Could you check a few things on this model? Use its own coordinates, in mm. A direction names the side the tool comes from. Give positions to 0.01 mm unless a question says otherwise; leave off trailing zeros. Write each loop counter-clockwise with the first axis right and the second up, starting at its lowest first coordinate (ties: lowest second). Pieces come first, ordered by that corner, then holes. Notation, with made-up numbers: (0, -38.5) - (9, -38.5) arc R11 ccw to (9, -26.5) - close; hole circle Ø7 at (-37.75, -24.5). An arc over 180 degrees is marked (long way). Use one line per item in the form item = value.
Autodesk Inventor part; units mm, degrees
ref_plane "YZ Plane" through (0, 0, 0) normal (1, 0, 0) x (0, 1, 0)
ref_plane "XZ Plane" through (0, 0, 0) normal (0, 1, 0) x (-1, 0, 0)
ref_plane "XY Plane" through (0, 0, 0) normal (0, 0, 1) x (1, 0, 0)
sketch "Skizze1" plane through (0, 0, 0) normal (0, 1, 0) x (-1, 0, 0)
  line L0 (0, 0) -> (54.1, 0)
  line L1 (54.1, 0) -> (54.1, -94.74)
  line L2 (54.1, -94.74) -> (0, -94.74)
  line L3 (0, -94.74) -> (0, 0)
  dimension "d0" = 94.74
  dimension "d1" = 54.1
extrude "Extrusion1" add sketch "Skizze1" along normal blind 1.5
sketch "Skizze2" plane through (0, 1.5, 0) normal (0, 1, 0) x (1, 0, 0)
  line L0 (-54.1, 0) -> (0, 0)
  line L1 (0, 94.74) -> (-54.1, 94.74)
  line L2 (0, 0) -> (-54.1, 0)
  line L3 (-54.1, 0) -> (-54.1, 94.74)
  line L4 (-54.1, 94.74) -> (0, 94.74)
  line L5 (0, 94.74) -> (0, 0)
  line L6 (-53.35, 93.99) -> (-53.35, 0.75)
  line L7 (-53.35, 0.75) -> (-0.75, 0.75)
  line L8 (-0.75, 0.75) -> (-0.75, 93.99)
  line L9 (-0.75, 93.99) -> (-53.35, 93.99)
  dimension "d4" = 0.75
extrude "Extrusion2" cut sketch "Skizze2" against normal blind 0.75
sketch "Skizze3" plane through (0, 1.5, 0) normal (0, 1, 0) x (1, 0, 0)
  circle A0 centre (-42.29, 9.27) radius 4
  circle A1 centre (-42.29, 85.47) radius 4
  circle A2 centre (-6.73, 85.47) radius 4
  circle A3 centre (-6.73, 9.27) radius 4
  line L0 (0, 0) -> (-54.1, 0)
  line L1 (-0.75, 0.75) -> (-0.75, 93.99)
  line L2 (-53.35, 0.75) -> (-0.75, 0.75)
  dimension "d7" = 8
  dimension "d8" = 8
  dimension "d9" = 8
  dimension "d10" = 8
  dimension "d12" = 5.98
  dimension "d13" = 5.98
  dimension "d14" = 35.56
  dimension "d15" = 35.56
  dimension "d16" = 8.52
  dimension "d17" = 76.2
extrude "Extrusion3" add sketch "Skizze3" along normal blind 4.25
sketch "Skizze4" plane through (-42.29, 5.75, -9.27) normal (0, 1, 0) x (1, 0, 0)
  circle A0 centre (0, 0) radius 4
  circle A1 centre (0, 0) radius 1.55
  circle A2 centre (35.56, 0) radius 4
  circle A3 centre (35.56, 0) radius 1.55
  circle A4 centre (35.56, 76.2) radius 4
  circle A5 centre (35.56, 76.2) radius 1.55
  circle A6 centre (0, 76.2) radius 4
  circle A7 centre (0, 76.2) radius 1.55
  point P0 (42.29, -9.27)
  dimension "d20" = 3.1
  dimension "d21" = 3.1
  dimension "d22" = 3.1
  dimension "d23" = 3.1
extrude "Extrusion4" cut sketch "Skizze4" against normal blind 10 contours A1 | A3 | A5 | A7
sketch "Skizze5" plane through (0, 0, 0) normal (0, -1, 0) x (1, 0, 0)
  circle A0 centre (-6.73, -9.27) radius 1.55
  circle A1 centre (-6.73, -9.27) radius 3
  circle A2 centre (-42.29, -9.27) radius 1.55
  circle A3 centre (-42.29, -9.27) radius 3
  circle A4 centre (-42.29, -85.47) radius 4
  circle A5 centre (-42.29, -85.47) radius 3
  circle A6 centre (-6.73, -85.47) radius 1.55
  circle A7 centre (-6.73, -85.47) radius 3
  point P0 (0, 0)
  dimension "d26" = 6
  dimension "d27" = 6
  dimension "d28" = 6
  dimension "d29" = 6
extrude "Extrusion5" cut sketch "Skizze5" against normal blind 3.5 contours A1 | A3 | A5 | A7
properties part number "Bottom"
1. Which directions (+Z, -Z, +X, -X, +Y, -Y) give clear straight access to the entire face, cutting with the end or side of a thin tool? Please do faces 1 (the face through (-40.8, 4.6, -9.7)), 2 (the face through (-44.671, 1.726, -87.295)), 3 (the face through (-40.14, 3.595, -5.897)).
Response values:
face_1 = +Y, -Y
face_2 = -Y
face_3 = +Y
2. For pin 1 (4 mm diameter, centred on x = -42.29, z = -85.47, fed in from -Y); pin 2 (0.8 mm diameter, centred on x = -25, y = 1.5, fed in from +Z); pin 3 (1.5 mm diameter, centred on x = -7.5, y = 3, fed in from +Z), each with a flat end and sliding along its axis, tell me the tip position at first contact or that it passes through.
Response values:
pin_1 = 3.5
pin_2 = -0.75
pin_3 = -5.27
3. If I drill on line 1 (Z direction, x = -42.29, y = 4.1); line 2 (X direction, y = 5.2, z = -85.47); line 3 (Z direction, x = -6.73, y = 1), over which ranges is the centre line in solid material (lowest first)? Write a range as from..to.
Response values:
line_1 = -89.47..-87.02, -83.92..-81.47, -13.27..-10.82, -7.72..-5.27
line_2 = -46.29..-43.84, -40.74..-38.29, -10.73..-8.28, -5.18..-2.73
line_3 = -93.99..-88.47, -82.47..-12.27, -6.27..-0.75
4. Imagine slicing it at A-A, the plane y = 2.5. List the corners of the cut face in (x, z) for me, and give its area (3 significant figures).
Response values:
outline = circle Ø8 at (-42.29, -85.47); circle Ø8 at (-42.29, -9.27); circle Ø8 at (-6.73, -85.47); circle Ø8 at (-6.73, -9.27); hole circle Ø6 at (-42.29, -85.47); hole circle Ø6 at (-42.29, -9.27); hole circle Ø6 at (-6.73, -85.47); hole circle Ø6 at (-6.73, -9.27)
area = 88.0 mm²
5. If we mould it in two halves opening along X, with no side actions, what happens to faces 4 (the face through (-5, 3.5, -87)), 5 (the face through (-7.251, 3.595, -5.304)), 6 (the face through (-42.3, 5.75, -7.5))? For each: pulls with the +X half, pulls with the -X half, needs draft (parallel to the pull), parting line crosses it, or undercut.
Response values:
face_4 = undercut
face_5 = undercut
face_6 = needs draft
6. Imagine slicing it at D-D, the plane x = -13. List the corners of the cut face in (y, z) for me, and give its area (3 significant figures).
Response values:
outline = (0, -94.74) - (0.75, -94.74) - (0.75, -93.99) - (1.5, -93.99) - (1.5, -0.75) - (0.75, -0.75) - (0.75, 0) - (0, 0) - close
area = 141 mm²
7. Imagine slicing it at B-B, the plane z = -85.47. State how many separate pieces and enclosed holes the cut face has, and give its area (3 significant figures).
Response values:
separate_pieces = 3
enclosed_holes = 0
area = 92.1 mm²
